from build123d import *

# Parameters (mm, degrees)
F1_DEPTH     = 11.43
F2_SIZE      = 5.08
F4_DEPTH     = 4.572
F5_T4_DEPTH  = 35.6101050897
F5_T9_DEPTH  = 44.6545724626
F5_T14_DEPTH = 36.379020654
F5_T19_DEPTH = 32.4730482843
F7_DEPTH     = 3.302
F8_T4_DEPTH  = 87.5344337201


# Not quite as in the source:
# - a fillet or chamfer that OpenCascade refuses, or shapes differently, is made with other operations: its cross-section is extruded or revolved along the edge and cut away or added


with BuildPart() as f1:
    # F0 (on Top) → F1 (new body)
    with BuildSketch(Plane.XY):
        Polygon((0, -46.853557229), (0, 64.6125674248), (-15.2085125446, 64.6125674248), (-20.4984303564, 26.6385115683), (-15.7752875239, 21.5375181288), (-20.4984303564, 13.9804948121), (-82.6549530029, 42.8861156106), (-82.6549530029, 20.5928906798), (-42.2248728573, -15.6808290631), (-24.276940152, -36.2737216055), align=None)
    extrude(amount=F1_DEPTH)

    # F2
    f2_edges = [f1.edges().sort_by_distance(p)[0] for p in [
        (-51.576692, 28.433305, 11.43),
        (-82.654953, 31.739503, 11.43),
        (-62.439913, 2.456031, 11.43),
        (-18.136859, 17.759006, 11.43),
        (-18.136859, 24.088015, 11.43),
        (-17.853471, 45.625539, 11.43),
        (-7.604256, 64.612567, 11.43),
        (-33.250907, -25.977275, 11.43),
        (-12.13847, -41.563639, 11.43),
    ]]
    chamfer(f2_edges, length=F2_SIZE)

    # F3 (on face) → F4 (join)
    with BuildSketch(Plane.XY.offset(11.43)):
        Polygon((0, 22.1388745617), (0, 52.5213219225), (-8.6118569598, 48.5538840294), (-12.3903686181, 30.4170250893), (-6.3447491266, 22.1388745617), align=None)
    extrude(amount=F4_DEPTH)

    # F5: chamfer of 5.08 on 4 edges, made by hand


with BuildPart() as f5_tool2:
    # F5_s3 → F5_t4 (new body)
    with BuildSketch(Plane(origin=(31.8255199814, 14.6618522037, 0), x_dir=(0, 0, 1), z_dir=(-0.9082507089, -0.418426397, 0))):
        Polygon((10.922, 47.7025278707), (16.002, 42.6225278707), (16.002, 47.7025278707), align=None)
    extrude(amount=F5_T4_DEPTH)

    split(bisect_by=Plane.XY.offset(11.43), keep=Keep.TOP)


with BuildPart() as f1_1:
    add(f1.part)

    # F5_t1: cut F5_tool2
    add(f5_tool2.part, mode=Mode.SUBTRACT)


with BuildPart() as f5_tool7:
    # F5_s8 → F5_t9 (new body)
    with BuildSketch(Plane(origin=(12.0008759003, 57.6042137868, 0), x_dir=(0, 0, 1), z_dir=(-0.203954222, -0.9789804264, 0))):
        Polygon((10.922, 18.3336090407), (16.002, 13.2536090407), (16.002, 18.3336090407), align=None)
    extrude(amount=F5_T9_DEPTH)

    split(bisect_by=Plane.XY.offset(11.43), keep=Keep.TOP)


with BuildPart() as f1_2:
    add(f1_1.part)

    # F5_t6: cut F5_tool7
    add(f5_tool7.part, mode=Mode.SUBTRACT)


with BuildPart() as f5_tool12:
    # F5_s13 → F5_t14 (new body)
    with BuildSketch(Plane(origin=(-26.5018256682, 36.2884403239, 0), x_dir=(0, 0, 1), z_dir=(0.5897750216, -0.8075675971, 0))):
        Polygon((10.922, -7.9331414154), (16.002, -13.0131414154), (16.002, -7.9331414154), align=None)
    extrude(amount=F5_T14_DEPTH)

    split(bisect_by=Plane.XY.offset(11.43), keep=Keep.TOP)


with BuildPart() as f1_3:
    add(f1_2.part)

    # F5_t11: cut F5_tool12
    add(f5_tool12.part, mode=Mode.SUBTRACT)


with BuildPart() as f5_tool17:
    # F5_s18 → F5_t19 (new body)
    with BuildSketch(Plane.YZ.offset(-19.4088987055)):
        Polygon((22.1388745617, 10.922), (27.2188745617, 16.002), (22.1388745617, 16.002), align=None)
    extrude(amount=F5_T19_DEPTH)

    split(bisect_by=Plane.XY.offset(11.43), keep=Keep.TOP)


with BuildPart() as f1_4:
    add(f1_3.part)

    # F5_t16: cut F5_tool17
    add(f5_tool17.part, mode=Mode.SUBTRACT)

    # F6 (on face) → F7 (join)
    with BuildSketch(Plane.XY.offset(11.43)):
        Polygon((-4.4554928318, -2.4560331367), (0, 14.7361988202), (-6.8530052353, 0), (-74.3786075584, 31.4024879744), (-74.3786075584, 27.9609914869), (-6.8530052353, -12.1079402775), align=None)
    extrude(amount=F7_DEPTH)

    # F8: chamfer of 5.08 on 1 edges, made by hand


with BuildPart() as f8_tool2:
    # F8_s3 → F8_t4 (new body)
    with BuildSketch(Plane(origin=(-5.6344557861, 2.6202791827, 0), x_dir=(0, 0, 1), z_dir=(-0.9067455979, 0.4216781007, 0))):
        Polygon((9.652, -2.8897622316), (14.732, -7.9697622316), (14.732, -2.8897622316), align=None)
    extrude(amount=F8_T4_DEPTH)

    split(bisect_by=Plane.XY.offset(11.43), keep=Keep.TOP)


with BuildPart() as f1_5:
    add(f1_4.part)

    # F8_t1: cut F8_tool2
    add(f8_tool2.part, mode=Mode.SUBTRACT)


solid = f1_5.part
Source: CAD feature listing. Evaluate the final solid. Frame: model axes, mm. A direction names the side the tool comes from. Give positions to 0.01 mm unless a question says otherwise; leave off trailing zeros. Order: outer loops, then holes, each group sorted by start corner. A loop starts at its lowest first (then second) coordinate and runs counter-clockwise, first axis right, second up. Notation, with made-up numbers: (-27.75, -5.75) -> (0.25, -5.75) arc R13 ccw to (0.25, -1.75) -> close; hole circle Ø6 at (-9.75, 29.5). An arc over 180 degrees is marked (long way). Write item = value, one per line.
Q1. Cut plane C-C, the plane x = -65.5. Output: boundary loops of the cut face in (y, z), and give its area (3 significant figures).
Data:
outline = (5.2, 0) -> (34.91, 0) -> (34.91, 6.35) -> (29.31, 11.43) -> (25.31, 11.43) -> (22.69, 13.81) -> (22.69, 11.43) -> (12.03, 11.43) -> (5.2, 6.35) -> close
area = 311 mm^2
Q2. Material intervals for line 1 (Z direction, x = -9, y = 20); line 2 (X direction, y = 56, z = 7); line 3 (X direction, y = 22, z = 9.5), sorted ascending. Write a range as from..to.
Data:
line_1 = 0..11.43
line_2 = -15.75..0
line_3 = -79.5..-45.21, -11.91..0
Q3. Pin query (flat end, axial travel): pin 1 (5 mm diameter, centred on x = -43, z = 11.5, fed in from +Y); pin 2 (1.1 mm diameter, centred on y = 28.5, z = 12.5, fed in from -X); pin 3 (8 mm diameter, centred on x = -55.5, z = 2, fed in from +Y). Return the tip coordinate at first contact, or that it passes through.
Data:
pin_1 = 21.76
pin_2 = -74.38
pin_3 = 32.12
Q4. Cut plane B-B, the plane z = 5. Output: boundary loops of the cut face in (x, y).
Data:
outline = (-82.65, 20.59) -> (-42.22, -15.68) -> (-24.28, -36.27) -> (0, -46.85) -> (0, 64.61) -> (-15.21, 64.61) -> (-20.5, 26.64) -> (-15.78, 21.54) -> (-20.5, 13.98) -> (-82.65, 42.89) -> close
Q5. Cut plane A-A, the plane y = 41. Output: boundary loops of the cut face in (x, z), and give its area (3 significant figures).
Data:
outline = (-82.65, 0) -> (-78.6, 0) -> (-78.6, 6.35) -> (-81.45, 7.55) -> (-82.65, 6.35) -> close; (-18.5, 0) -> (0, 0) -> (0, 16) -> (-5, 16) -> (-9.67, 11.43) -> (-13.37, 11.43) -> (-18.5, 6.35) -> close
area = 260 mm^2
Q6. Set-up query: faces 4 (the face through (-2.26, 6.02, 13.06)), 5 (the face through (-20, 0, 14.732)), 6 (the face through (-18.104, 17.812, 3.131)), 7 (the face through (-7.187, 27.975, 13.684)). Return all of +Z, -Z, +X, -X, +Y, -Y with unobstructed straight access to the full face (end or side cutting, diameter ignored); none if empty.
Data:
face_4 = +Z, +X, -Y
face_5 = +Z, +X, -X, -Y
face_6 = +Z, -Z
face_7 = +Z
Q7. Cut plane D-D, the plane y = -19. Output: boundary loops of the cut face in (x, z), and give its area (3 significant figures).
Data:
outline = (-39.33, 0) -> (0, 0) -> (0, 11.43) -> (-32.59, 11.43) -> (-39.33, 6.35) -> close
area = 432 mm^2
Q8. Pull-direction query (X, two-part tool) for faces 1 (the face through (-41.09, 8.21, 13.06)), 2 (the face through (0, 8, 6)), 3 (the face through (-51.14, 28.23, 3.13)); classes: released by +X, released by -X, zero draft, split by the parting line, or undercut.
Data:
face_1 = released by -X
face_2 = released by +X
face_3 = undercut
